Source: CAD feature listing. Evaluate the final solid. Frame: model axes, mm. Face numbers are marked on the shaded views. A direction names the side the tool comes from. Give positions to 0.01 mm unless a question says otherwise; leave off trailing zeros. Loops run counter-clockwise (first coordinate to the right, second up) from the corner with the lowest first, then second, coordinate; pieces in that order, holes last. Notation, with made-up numbers: (-35.5, 5) -> (-7.5, 5) arc R31 cw to (-7.5, 44) -> close; hole circle Ø1 at (-29, 9.5). An arc over 180 degrees is marked (long way). Answer as a JSON object with one key per item and string values. Group by question number.
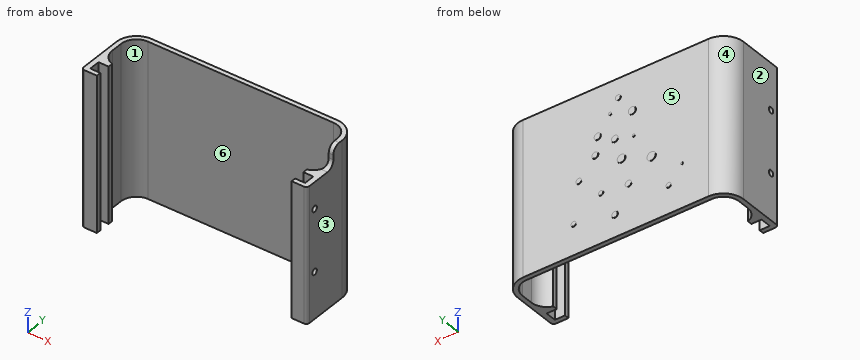
from build123d import *

# Parameters (mm, degrees)
BOSS_EXTRUDE1_DEPTH = 100
SKETCH2_R           = 1.925
CUT_EXTRUDE1_DEPTH  = 181.013888353
SKETCH3_W           = 10
SKETCH3_H           = 22.639392014
CUT_EXTRUDE2_DEPTH  = 13
FILLET1_R           = 5
SKETCH4_R           = 1.733173836
SKETCH4_R_2         = 0.981586666
SKETCH4_R_3         = 2.392571232
SKETCH4_R_4         = 2.109303231
SKETCH4_R_5         = 2.027090755
SKETCH4_R_6         = 2.155813145
SKETCH4_R_7         = 2.801748037
SKETCH4_R_8         = 1.588123218
SKETCH4_R_9         = 1.944759062
SKETCH4_R_10        = 2.597034209
SKETCH4_R_11        = 0.847315687
SKETCH4_R_12        = 1.785604619
SKETCH4_R_13        = 1.51506652
SKETCH4_R_14        = 2.019517128
SKETCH4_R_15        = 0.753353873
BOSS_EXTRUDE2_DEPTH = 0.2


with BuildPart() as part:
    # Sketch1 → Boss-Extrude1 (new body)
    with BuildSketch(Plane.XY):
        with BuildLine():
            Line((-63, -7.1), (-63, -10.1))
            Line((-63, -10.1), (-71, -10.1))
            ThreePointArc((-71, -10.1), (-72.414213562, -9.514213562), (-73, -8.1))
            Line((-73, -8.1), (-73, 20))
            ThreePointArc((-73, 20), (-69.192388155, 29.192388155), (-60, 33))
            Line((-60, 33), (60, 33))
            ThreePointArc((60, 33), (69.192388155, 29.192388155), (73, 20))
            Line((73, 20), (73, -8.1))
            ThreePointArc((73, -8.1), (72.414213562, -9.514213562), (71, -10.1))
            Line((71, -10.1), (63, -10.1))
            Line((63, -10.1), (63, -7.1))
            Line((63, -7.1), (69.5, -7.1))
            Line((69.5, -7.1), (69.5, 0))
            Line((69.5, 0), (63, 0))
            Line((63, 0), (63, 3))
            ThreePointArc((63, 3), (68.062257748, 6.623312231), (70, 12.539392014))
            Line((70, 12.539392014), (70, 20))
            ThreePointArc((70, 20), (67.071067812, 27.071067812), (60, 30))
            Line((60, 30), (-60, 30))
            ThreePointArc((-60, 30), (-67.071067812, 27.071067812), (-70, 20))
            Line((-70, 20), (-70, 12.539392014))
            ThreePointArc((-70, 12.539392014), (-68.062257748, 6.623312231), (-63, 3))
            Line((-63, 3), (-63, 0))
            Line((-63, 0), (-69.5, 0))
            Line((-69.5, 0), (-69.5, -7.1))
            Line((-69.5, -7.1), (-63, -7.1))
        make_face()
    extrude(amount=BOSS_EXTRUDE1_DEPTH)

    # Sketch2 → Cut-Extrude1 (cut, through all)
    with BuildSketch(Plane(origin=(73, 0, 0), x_dir=(0, 0, -1), z_dir=(1, 0, 0))):
        with Locations((-70, -3.55)):
            Circle(SKETCH2_R)
        with Locations((-30, -3.55)):
            Circle(SKETCH2_R)
    extrude(amount=-CUT_EXTRUDE1_DEPTH, mode=Mode.SUBTRACT)

    # Sketch3 → Cut-Extrude2 (cut)
    with BuildSketch(Plane.XY.offset(100)):
        with Locations((68, 1.219696007)):
            Rectangle(SKETCH3_W, SKETCH3_H)
    extrude(amount=-CUT_EXTRUDE2_DEPTH, mode=Mode.SUBTRACT)

    # Fillet1
    # the kernel refuses this fillet: 5 mm, written as the material it adds along each edge
    with BuildSketch(Plane(origin=(57.5, 12.539392014, 87), x_dir=(0, 0, 1), z_dir=(1, 0, 0))) as fillet1_piece_1_section:
        with BuildLine():
            CenterArc((FILLET1_R, FILLET1_R), FILLET1_R, 180, 90)
            Line((0, FILLET1_R), (0, 0))
            Line((0, 0), (FILLET1_R, 0))
        make_face()
    fillet1_piece_1 = extrude(amount=15.5, mode=Mode.PRIVATE)
    fillet1_piece_1 = fillet1_piece_1 - Plane(origin=(60, 12.539392014, 87.300010579), x_dir=(0.30000000000000276, -0.9539392014169449, 0), z_dir=(0, 0, -1)) * Cylinder(10, 52, mode=Mode.PRIVATE)
    add(fillet1_piece_1)
    # the kernel refuses this fillet: 5 mm, written as the material it takes off along each edge
    with BuildSketch(Plane(origin=(57.5, 12.539392014, 100), x_dir=(0, 1, 0), z_dir=(1, 0, 0))) as fillet1_2_piece_1:
        with BuildLine():
            CenterArc((FILLET1_R, -FILLET1_R), FILLET1_R, 90, 90)
            Line((0, -FILLET1_R), (0, 0))
            Line((0, 0), (FILLET1_R, 0))
        make_face()
    extrude(amount=28, mode=Mode.SUBTRACT)

    # Sketch4 → Boss-Extrude2 (add)
    with BuildSketch(Plane(origin=(0, 33, 0), x_dir=(1, 0, 0), z_dir=(0, 1, 0))):
        with Locations(Location((-1.621353912, -87.688909541, 0), (0, 0, 90))):
            Circle(SKETCH4_R)
        with Locations(Location((3.597208545, -79.608554769, 0), (0, 0, 90))):
            Circle(SKETCH4_R_2)
        with Locations(Location((-10.711753031, -75.568377383, 0), (0, 0, 90))):
            Circle(SKETCH4_R_3)
        with Locations(Location((0.487949319, -62.457213607, 0), (0, 0, 90))):
            Circle(SKETCH4_R_4)
        with Locations(Location((13.192629836, -57.387579146, 0), (0, 0, 90))):
            Circle(SKETCH4_R_5)
        with Locations(Location((11.615509985, -68.68582041, 0), (0, 0, 90))):
            Circle(SKETCH4_R_6)
        with Locations(Location((-23.168966637, -41.226869603, 0), (0, 0, 90))):
            Circle(SKETCH4_R_7)
        with Locations(Location((-34.279454449, -18.164190358, 0), (0, 0, 90))):
            Circle(SKETCH4_R_8)
        with Locations(Location((0.487949319, -14.292353696, 0), (0, 0, 90))):
            Circle(SKETCH4_R_9)
        with Locations(Location((27.164909963, -19.752313576, 0), (0, 0, 90))):
            Circle(SKETCH4_R_8)
        with Locations(Location((-3.730657143, -48.128839304, 0), (0, 0, 90))):
            Circle(SKETCH4_R_10)
        with Locations(Location((-11.721797377, -59.414669901, 0), (0, 0, 90))):
            Circle(SKETCH4_R_11)
        with Locations(Location((23.798095474, -45.531805095, 0), (0, 0, 90))):
            Circle(SKETCH4_R_12)
        with Locations(Location((9.489133899, -31.799789035, 0), (0, 0, 90))):
            Circle(SKETCH4_R_13)
        with Locations(Location((-8.319181799, -30.284722516, 0), (0, 0, 90))):
            Circle(SKETCH4_R_14)
        with Locations(Location((-42.864831394, -28.265205387, 0), (0, 0, 90))):
            Circle(SKETCH4_R_15)
    extrude(amount=BOSS_EXTRUDE2_DEPTH)


solid = part.part
(1) Section query C-C on y = 5.5. Return the cut outline in (x, z), plus the area to 3 significant figures.
(2) Section query B-B on z = 24.5. Return the cut outline in (x, y), plus the area to 3 significant figures.
(3) Section query A-A on y = -3.55. Return the cut outline in (x, z) (3 decimals), plus the area to 3 significant figures.
(4) Access query for the marked faces 4, 5 and 6. Directions: +Z, -Z, +X, -X, +Y, -Y. A direction counts if a zero-diameter tool reaches every point of the face in a straight line with its end or side. Return the directions, or none.
(5) Mould query, pull axis X, two halves, no side actions, for the marked faces 1, 2 and 3. Classes: pulls with the +X half, pulls with the -X half, needs draft (parallel to the pull), parting line crosses it, or undercut.
(6) First-contact query: pin 1 (1 mm diameter, centred on x = -36.5, z = 53.5, fed in from -Y); pin 2 (1.5 mm diameter, centred on x = 71.5, z = 93, fed in from -Y); pin 3 (3 mm diameter, centred on x = -53, z = 83.5, fed in from +Y); pin 4 (3 mm diameter, centred on y = -3.55, z = 70, fed in from +X). Flat tips, straight axial feed; report the tip coordinate or a pass-through.
(7) Material intervals for line 1 (X direction, y = 9.5, z = 43); line 2 (X direction, y = 20.5, z = 93); line 3 (Y direction, x = -67, z = 51), sorted ascending. Write a range as from..to.
(8) Section query D-D on x = -47. Return the cut outline in (y, z), plus the area to 3 significant figures.
Result:
{
 "1": {"outline": "(-73, 0) -> (-67.1, 0) -> (-67.1, 100) -> (-73, 100) -> close; (67.1, 0) -> (73, 0) -> (73, 87) -> (67.1, 87) -> close", "area": "1,100 mm²"},
 "2": {"outline": "(-73, -8.1) arc R2 ccw to (-71, -10.1) -> (-63, -10.1) -> (-63, -7.1) -> (-69.5, -7.1) -> (-69.5, 0) -> (-63, 0) -> (-63, 3) arc R10 cw to (-70, 12.54) -> (-70, 20) arc R10 cw to (-60, 30) -> (60, 30) arc R10 cw to (70, 20) -> (70, 12.54) arc R10 cw to (63, 3) -> (63, 0) -> (69.5, 0) -> (69.5, -7.1) -> (63, -7.1) -> (63, -10.1) -> (71, -10.1) arc R2 ccw to (73, -8.1) -> (73, 20) arc R13 ccw to (60, 33) -> (-60, 33) arc R13 ccw to (-73, 20) -> close", "area": "774 mm²"},
 "3": {"outline": "(-73, 0) -> (-69.5, 0) -> (-69.5, 28.075) -> (-73, 28.075) -> close; (-73, 31.925) -> (-69.5, 31.925) -> (-69.5, 68.075) -> (-73, 68.075) -> close; (-73, 71.925) -> (-69.5, 71.925) -> (-69.5, 100) -> (-73, 100) -> close; (69.5, 0) -> (73, 0) -> (73, 28.075) -> (69.5, 28.075) -> close; (69.5, 31.925) -> (73, 31.925) -> (73, 68.075) -> (69.5, 68.075) -> close; (69.5, 71.925) -> (73, 71.925) -> (73, 87) -> (69.5, 87) -> close", "area": "601 mm²"},
 "4": {"face 4": "+Z, -Z, -X, +Y", "face 5": "+Y", "face 6": "+Z, -Z, -Y"},
 "5": {"face 1": "undercut", "face 2": "pulls with the -X half", "face 3": "pulls with the +X half"},
 "6": {"pin 1": "y = 30", "pin 2": "y = 12.54", "pin 3": "y = 33", "pin 4": "through"},
 "7": {"line 1": "-73..-69.53, 69.53..73", "line 2": "-72.99..-69.99, 69.99..72.99", "line 3": "-10.1..-7.1, 0..5.4, 27.14..30.95"},
 "8": {"outline": "(30, 0) -> (33, 0) -> (33, 100) -> (30, 100) -> close", "area": "300 mm²"}
}
